For this review, use the dimensioned drawing (mm, ordinates from the lowest corner) and the shaded views. A direction names the side the tool comes from. Round coordinates to 2 decimals unless told otherwise and drop trailing zeros. Order: outer loops, then holes, each group sorted by start corner. A loop starts at its lowest first (then second) coordinate and runs counter-clockwise, first axis right, second up. Notation, with made-up numbers: M 68,64.25 L 122,64.25 A9 cw 122,71.25 Z; hole C 8.5,51.25 d4. An arc over 180 degrees is marked long. Use a Markdown table: item, result. Add a question column.
1. Consider section A-A on y = 12.7. State the section outline as (x, z) points, then the cut area to 3 significant figures.
2. Consider section C-C on x = 12.7. State the section outline as (y, z) points.
3. Consider section D-D on z = 8.5. State the section outline as (x, y) points.
4. Insertion check: P1, Ø1, axis at x = 5, y = 9.5, coming from the +Z side; P2, Ø14, axis at y = 11, z = 111.5, coming from the -X side; P3, Ø2, axis at y = 16.5, z = 90, coming from the +X side. Each pin has a flat end and moves straight along its axis. Give the tip position at first contact, or say it passes through.
5. For the marked faces 1, 2 and 3, list the 3-axis set-ups (+Z, -Z, +X, -X, +Y, -Y) from which the entire face can be reached by the end or side of a thin tool; tool diameter is ignored.
6. To check wall thickness, follow probe 1 along Z at (x, y) = (11.5, 12.7); probe 2 along Z at (x, y) = (18.5, 9.75); probe 3 along X at (y, z) = (14, 90.5). State the ranges of each line that lie inside material, in increasing order.
7. Consider section B-B on z = 105. State the section outline as (x, y) points.
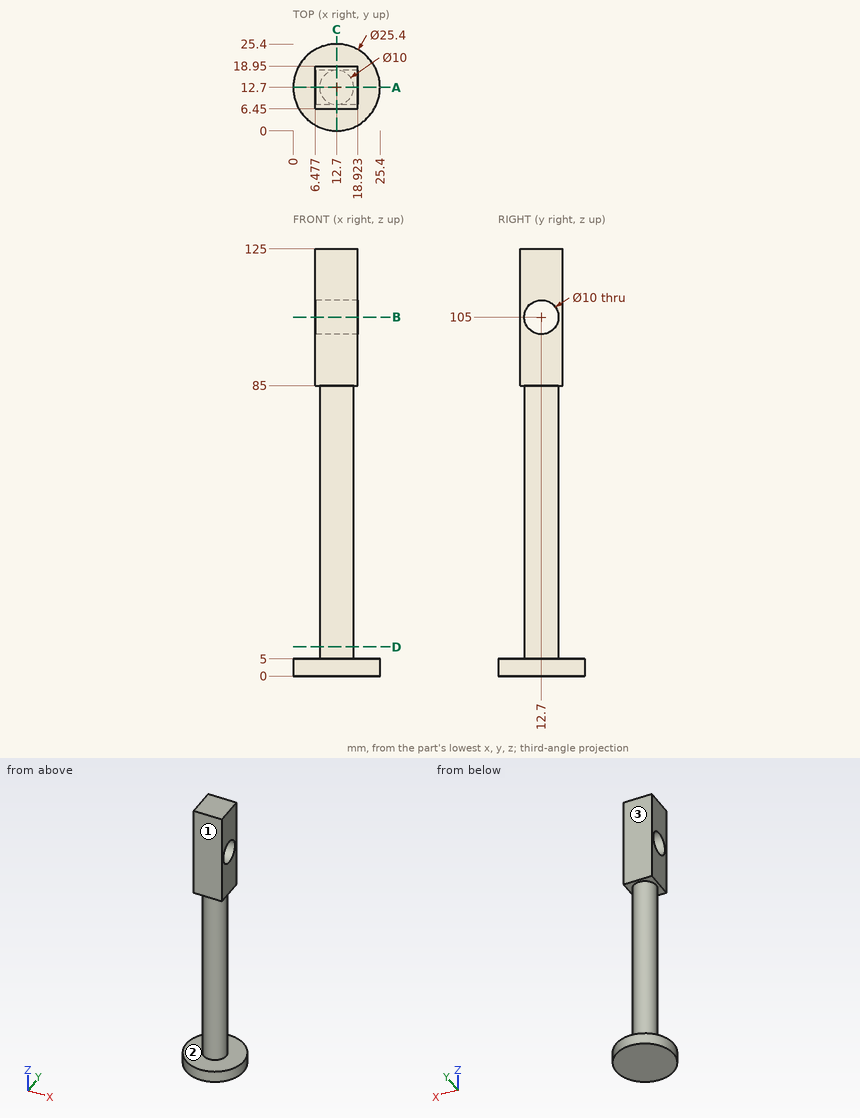
Answer block:
| question | item | result |
|---|---|---|
| 1 | outline | M 0,0 L 25.4,0 L 25.4,5 L 17.7,5 L 17.7,85 L 18.92,85 L 18.92,100 L 6.48,100 L 6.48,85 L 7.7,85 L 7.7,5 L 0,5 Z; M 6.48,110 L 18.92,110 L 18.92,125 L 6.48,125 Z |
| 1 | area | 1,300 mm^2 |
| 2 | outline | M 0,0 L 25.4,0 L 25.4,5 L 17.7,5 L 17.7,85 L 18.95,85 L 18.95,125 L 6.45,125 L 6.45,85 L 7.7,85 L 7.7,5 L 0,5 Z; hole C 12.7,105 d10 |
| 3 | outline | C 12.7,12.7 d10 |
| 4 | P1 | z = 5 |
| 4 | P2 | x = 6.48 |
| 4 | P3 | x = 18.92 |
| 5 | face 1 | +Z, +X, -X, -Y |
| 5 | face 2 | none |
| 5 | face 3 | +Z, +X, -X, +Y |
| 6 | probe 1 | 0 to 100, 110 to 125 |
| 6 | probe 2 | 0 to 5, 85 to 100.96, 109.04 to 125 |
| 6 | probe 3 | 6.48 to 18.92 |
| 7 | outline | M 6.48,6.45 L 18.92,6.45 L 18.92,7.7 L 6.48,7.7 Z; M 6.48,17.7 L 18.92,17.7 L 18.92,18.95 L 6.48,18.95 Z |
